Could you check a few things on this model? Use its own coordinates, in mm. A direction names the side the tool comes from. Round coordinates to 2 decimals unless told otherwise and drop trailing zeros. Loops run counter-clockwise (first coordinate to the right, second up) from the corner with the lowest first, then second, coordinate; pieces in that order, holes last.
from build123d import *

# Parameters (mm, degrees)
SKETCH_W        = 21.45
SKETCH_H        = 21.45
SKETCH_W_2      = 13.45
SKETCH_H_2      = 13.45
PAD_DEPTH       = 20
SKETCH001_W     = 21.45
SKETCH001_H     = 20
PAD001_DEPTH    = 15
POCKET_DEPTH    = 21.451
POCKET001_DEPTH = 21.451
CHAMFER_SIZE    = 2
CHAMFER001_SIZE = 5


with BuildPart() as part:
    # Sketch → Pad (new body)
    with BuildSketch(Plane.XY):
        Rectangle(SKETCH_W, SKETCH_H)
        Rectangle(SKETCH_W_2, SKETCH_H_2, mode=Mode.SUBTRACT)
    extrude(amount=PAD_DEPTH)

    # Sketch001 (on Face3 of Pad) → Pad001 (join)
    with BuildSketch(Plane.XZ.offset(10.725)):
        with Locations((0, 10)):
            Rectangle(SKETCH001_W, SKETCH001_H)
    extrude(amount=PAD001_DEPTH)

    # Sketch002 (on Face6 of Pad001) → Pocket (cut, through all)
    with BuildSketch(Plane(origin=(-10.725, 0, 0), x_dir=(0, -1, 0), z_dir=(-1, 0, 0))):
        Polygon((18.225, 11.5), (25.725, 11.5), (25.725, 8.5), (18.225, 8.5), (18.225, 4), (10.725, 4), (10.725, 16), (18.225, 16), align=None)
    extrude(amount=-POCKET_DEPTH, mode=Mode.SUBTRACT)

    # Sketch003 (on Face2 of Pocket) → Pocket001 (cut, through all)
    with BuildSketch(Plane(origin=(-10.725, 0, 0), x_dir=(0, -1, 0), z_dir=(-1, 0, 0))):
        with BuildLine():
            ThreePointArc((1.7, 15), (0, 16.7), (-1.7, 15))
            Line((-1.7, 15), (-1.7, 5))
            ThreePointArc((-1.7, 5), (0, 3.3), (1.7, 5))
            Line((1.7, 15), (1.7, 5))
        make_face()
    extrude(amount=-POCKET001_DEPTH, mode=Mode.SUBTRACT)

    # Chamfer
    chamfer_edges = [part.edges().sort_by_distance(p)[0] for p in [
        (-10.725, -1.7, 10),
        (-10.725, 1.7, 10),
        (-10.725, 0, 3.3),
        (-10.725, 0, 16.7),
        (10.725, 1.7, 10),
        (10.725, -1.7, 10),
        (10.725, 0, 3.3),
        (10.725, 0, 16.7),
    ]]
    chamfer(chamfer_edges, length=CHAMFER_SIZE)

    # Chamfer001
    chamfer001_edges = [part.edges().sort_by_distance(p)[0] for p in [
        (0, -25.725, 0),
        (0, -25.725, 20),
    ]]
    chamfer(chamfer001_edges, length=CHAMFER001_SIZE)


solid = part.part
Item 1: If we section it at C-C, the plane z = 12.75: Please give me the cut outline in (x, y) (3 decimals), then the cut area to 3 significant figures.
Results list:
outline: (-10.725, -25.725) - (10.725, -25.725) - (10.725, -18.225) - (-10.725, -18.225) - close; (-10.725, -10.725) - (10.725, -10.725) - (10.725, -3.7) - (8.725, -1.7) - (6.725, -1.7) - (6.725, -6.725) - (-6.725, -6.725) - (-6.725, -1.7) - (-8.725, -1.7) - (-10.725, -3.7) - close; (-10.725, 3.7) - (-8.725, 1.7) - (-6.725, 1.7) - (-6.725, 6.725) - (6.725, 6.725) - (6.725, 1.7) - (8.725, 1.7) - (10.725, 3.7) - (10.725, 10.725) - (-10.725, 10.725) - close
area: 405 mm2
Item 2: If I drill on line 1 along Y through (x, z) = (-2.5, 12.5) (3 decimals); line 2 along X through (y, z) = (6.5, 1.5) (3 decimals), over which ranges is the centre line in solid material (lowest first)?
Results list:
line 1: y = -25.725 to -18.225, -10.725 to -6.725, 6.725 to 10.725
line 2: x = -10.725 to -6.725, 6.725 to 10.725
Item 3: Will these pins go through, and if not, where does the flat tip stop? pin 1 (2 mm diameter, centred on x = 5, y = -22.5, fed in from -Z) (3 decimals); pin 2 (1 mm diameter, centred on y = 1.5, z = 7.5, fed in from +X) (3 decimals).
Results list:
pin 1: stops at z = 0.775
pin 2: stops at x = 9.025
Item 4: If we section it at B-B, the plane y = 0: Please give me the cut outline in (x, z) (3 decimals), then the cut area to 3 significant figures.
Results list:
outline: (-10.725, 0) - (-6.725, 0) - (-6.725, 3.3) - (-8.725, 3.3) - (-10.725, 1.3) - close; (-10.725, 18.7) - (-8.725, 16.7) - (-6.725, 16.7) - (-6.725, 20) - (-10.725, 20) - close; (6.725, 0) - (10.725, 0) - (10.725, 1.3) - (8.725, 3.3) - (6.725, 3.3) - close; (6.725, 16.7) - (8.725, 16.7) - (10.725, 18.7) - (10.725, 20) - (6.725, 20) - close
area: 44.8 mm2
Item 5: For faces 1 (the flat face through (6.725, -3, 10)), 2 (the conical face through (-9.267, -0.049, 2.759)), 3 (the conical face through (9.267, -0.049, 17.241)), 4 (the flat face through (8, -1.7, 10)), which set-ups out of +Z, -Z, +X, -X, +Y, -Y let a thin tool reach every point of the face, with its end or its side?
Results list:
face 1: +Z, -Z
face 2: -X
face 3: +X
face 4: +X, -X
Item 6: We'd pull the mould along Z, two halves only. Please class faces 5 (the flat face through (0, -25.725, 7)), 6 (the flat face through (0, -8, 0)), 7 (the cylindrical face through (7.7, 0, 16.7)), 8 (the flat face through (0, -15, 4)): released by +Z, released by -Z, zero draft, split by the parting line, or undercut.
Results list:
face 5: zero draft
face 6: released by -Z
face 7: undercut
face 8: undercut
Item 7: If we section it at D-D, the plane y = 5.5: Please give me the cut outline in (x, z) (3 decimals), then the cut area to 3 significant figures.
Results list:
outline: (-10.725, 0) - (-6.725, 0) - (-6.725, 20) - (-10.725, 20) - close; (6.725, 0) - (10.725, 0) - (10.725, 20) - (6.725, 20) - close
area: 160 mm2
Item 8: If we section it at A-A, the plane x = 3.75: Please give me the cut outline in (y, z) (3 decimals), then the cut area to 4 significant figures.
Results list:
outline: (-25.725, 5) - (-20.725, 0) - (-6.725, 0) - (-6.725, 20) - (-20.725, 20) - (-25.725, 15) - (-25.725, 11.5) - (-18.225, 11.5) - (-18.225, 16) - (-10.725, 16) - (-10.725, 4) - (-18.225, 4) - (-18.225, 8.5) - (-25.725, 8.5) - close; (6.725, 0) - (10.725, 0) - (10.725, 20) - (6.725, 20) - close
area: 322.5 mm2
